Check sheet for the modelled part. Datum: model origin and axes. Units: mm. Face numbers are marked on the shaded views. A direction names the side the tool comes from. Coordinates: 2 decimals unless noted, no trailing zeros. Loops run counter-clockwise (first coordinate to the right, second up) from the corner with the lowest first, then second, coordinate; pieces in that order, holes last. Notation, with made-up numbers: (10, 53) - (48, 53) arc R31 cw to (48, 81) - close; hole circle Ø4 at (1, -10). An arc over 180 degrees is marked (long way). Use a Markdown table: item, result. Add a question column.
1) Sectioned sample at A-A, the plane x = -31. Enter the section's corners in (y, z).
2) Sectioned sample at B-B, the plane y = -123. Enter the section's corners in (x, z), then the cut area to 3 significant figures.
3) Sectioned sample at C-C, the plane x = -3. Enter the section's corners in (y, z), then the cut area to 3 significant figures.
4) Sectioned sample at D-D, the plane z = -12.5. Enter the section's corners in (x, y), then the cut area to 3 significant figures.
5) Thickness scan on line 1 (Z direction, x = 14, y = -49); line 2 (X direction, y = -54, z = -19.5); line 3 (X direction, y = -217, z = -25). Record the ranges inside material, lowest first.
6) Go/stop test with flat-tipped pins: P1, Ø3, axis at y = -217, z = 18.5, coming from the +X side; P2, Ø6, axis at y = -94.5, z = -62, coming from the +X side; P3, Ø3, axis at y = -107.5, z = 27.5, coming from the +X side. Record where each tip stops, or that it passes through.
7) Tool access check on the marked faces 1, 2 and 3. Record the directions out of +Z, -Z, +X, -X, +Y, -Y that give a thin tool (end or side, any length) a straight path to the whole face; none if there is none.
from build123d import *

# Parameters (mm, degrees)
F1_DEPTH = 254


with BuildPart() as f1:
    # F0 (on Front) → F1 (new body)
    with BuildSketch(Plane.XZ):
        with BuildLine():
            Line((36.874757, 42.862148), (-43.897243, 42.862148))
            Line((-43.897243, 42.862148), (-43.897243, 34.099148))
            Line((-43.897243, 34.099148), (-7.067243, 34.099148))
            ThreePointArc((-7.067243, 34.099148), (5.195877, -16.827852), (-7.067243, -67.754852))
            Line((-7.067243, -67.754852), (-43.897243, -67.754852))
            Line((-43.897243, -67.754852), (-43.897243, -76.517852))
            Line((-43.897243, -76.517852), (36.874757, -76.517852))
            Line((36.874757, -76.517852), (36.874757, -67.754852))
            Line((36.874757, -67.754852), (0.044757, -67.754852))
            ThreePointArc((0.044757, -67.754852), (11.944951, -16.827852), (0.044757, 34.099148))
            Line((0.044757, 34.099148), (36.874757, 34.099148))
            Line((36.874757, 34.099148), (36.874757, 42.862148))
        make_face()
    extrude(amount=F1_DEPTH)


solid = f1.part
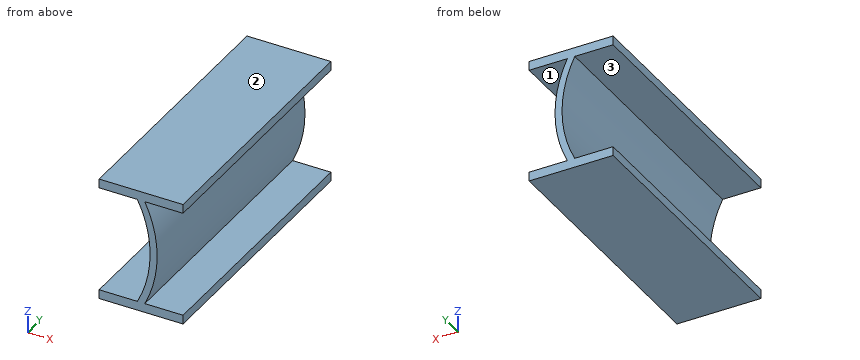
Solved:
| question | item | result |
|---|---|---|
| 1 | outline | (-254, -76.52) - (0, -76.52) - (0, -67.75) - (-254, -67.75) - close; (-254, 34.1) - (0, 34.1) - (0, 42.86) - (-254, 42.86) - close |
| 2 | outline | (-43.9, -76.52) - (36.87, -76.52) - (36.87, -67.75) - (0.04, -67.75) arc R114.92 ccw to (0.04, 34.1) - (36.87, 34.1) - (36.87, 42.86) - (-43.9, 42.86) - (-43.9, 34.1) - (-7.07, 34.1) arc R111.88 cw to (-7.07, -67.75) - (-43.9, -67.75) - close |
| 2 | area | 2,110 mm2 |
| 3 | outline | (-254, -76.52) - (0, -76.52) - (0, -58.86) - (-254, -58.86) - close; (-254, 25.2) - (0, 25.2) - (0, 42.86) - (-254, 42.86) - close |
| 3 | area | 8,970 mm2 |
| 4 | outline | (5.11, -254) - (11.86, -254) - (11.86, 0) - (5.11, 0) - close |
| 4 | area | 1,710 mm2 |
| 5 | line 1 | z = -76.52 to -67.75, 34.1 to 42.86 |
| 5 | line 2 | x = 5.16 to 11.91 |
| 5 | line 3 | x = 4.9 to 11.65 |
| 6 | P1 | stops at x = 6.85 |
| 6 | P2 | stops at x = 3.93 |
| 6 | P3 | stops at x = 3.67 |
| 7 | face 1 | +X, +Y, -Y |
| 7 | face 2 | +Z, +X, -X, +Y, -Y |
| 7 | face 3 | -X, +Y, -Y |
